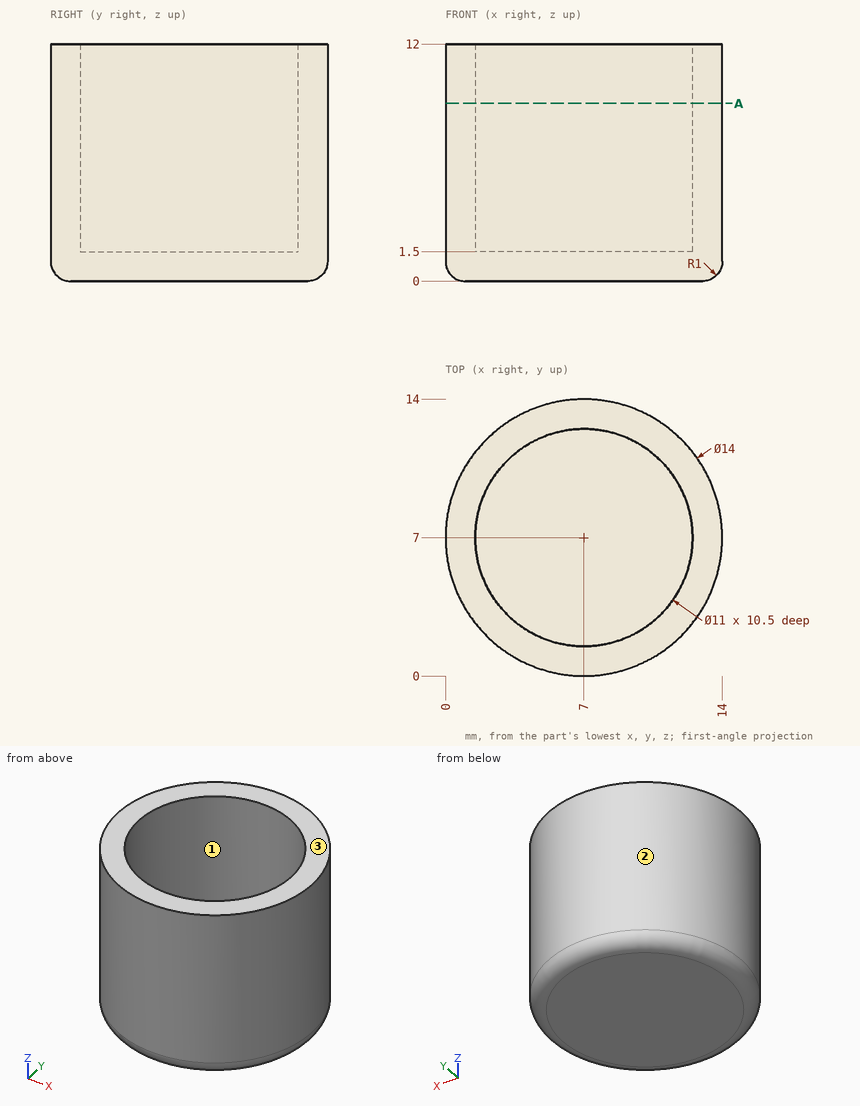
Design review of the part shown in the three views and the two pictorial views. Dimensions are in mm from the part's minimum x, y and z. Round coordinates to 2 decimals unless told otherwise and drop trailing zeros. Write each loop counter-clockwise with the first axis right and the second up, starting at its lowest first coordinate (ties: lowest second). Pieces come first, ordered by that corner, then holes.
Item 1: Clearance check with flat-ended pins moving along their axes: pin 1 Ø6 at (y, z) = (3, 8) entering from -X; pin 2 Ø2 at (y, z) = (4, 1.5) entering from +X; pin 3 Ø4 at (x, z) = (10.5, 2.5) entering from -Y; pin 4 Ø6 at (x, z) = (4, 10.5) entering from +Y. State where each tip first meets the part, or that it passes through.
Item 2: For probe 1 along Y at (x, z) = (7, 9.5); probe 2 along X at (y, z) = (4.75, 11.25); probe 3 along Z at (x, y) = (6, 7.25), list the stretches that pass through material, from the lowest coordinate up.
Item 3: The part is to be moulded in two halves that separate along X. For the marked faces 1, 2 and 3, say which applies: +X half, -X half, draft (parallel to the pull), parting line (faces both ways), or undercut.
Item 4: We need section A-A on z = 9. Write out the cut boundary in (x, y), and give its area (3 significant figures).
Returned:
1. pin 1: stops at x = 0.07
1. pin 2: stops at x = 13.71
1. pin 3: stops at y = 0.16
1. pin 4: stops at y = 14
2. probe 1: y = 0 to 1.5, 12.5 to 14
2. probe 2: x = 0.37 to 1.98, 12.02 to 13.63
2. probe 3: z = 0 to 1.5
3. face 1: undercut
3. face 2: parting line
3. face 3: draft
4. outline: circle Ø14 at (7, 7); hole circle Ø11 at (7, 7)
4. area: 58.9 mm2
